Can you work these out from the model? Positions are in its coordinate system, mm. A direction names the side the tool comes from. Round coordinates to 2 decimals unless told otherwise and drop trailing zeros. Write each loop counter-clockwise with the first axis right and the second up, starting at its lowest first coordinate (ties: lowest second). Pieces come first, ordered by that corner, then holes. Notation, with made-up numbers: M -3.5,45 L 24.5,45 A22 ccw 24.5,71 Z; hole C 68,73.5 d10. An arc over 180 degrees is marked long. Answer as a JSON object with one key per item and string values. Group by question number.
1) Suppose I cut it at C-C, the plane z = 111. Write out the boundary of the cut face in (x, y).
2) Please list where these lines run through material, in increasing order: L1, parallel to Z at x = 22, y = 16.5; L2, parallel to X at y = 1, z = 9.5. Write a range as [from, to].
3) Suppose I cut it at B-B, the plane y = 0. Write out the boundary of the cut face in (x, z).
4) On a 3-axis mill with a long thin cutter (end or side, diameter ignored), from which of +Z, -Z, +X, -X, +Y, -Y can I reach the whole of each face in a straight line? I mean faces 1 (the flat face through (0, 0, 148)), 2 (the flat face through (37, 0, 131)), 3 (the cylindrical face through (32.07, 0.9, 120.14)), 4 (the flat face through (17, 1, 143)). Say none if no direction works.
5) Suppose I cut it at D-D, the plane z = 132.5. Write out the boundary of the cut face in (x, y), and give its area (3 significant figures).
6) Suppose I cut it at A-A, the plane x = 0. Write out the boundary of the cut face in (y, z), and give its area (3 significant figures).
7) I'm going to push flat-ended pins straight in: pin 1 Ø3 at (x, y) = (31, -3.5) entering from +Z; pin 2 Ø3 at (y, z) = (29.5, 97.5) entering from +X; pin 3 Ø10 at (y, z) = (-11.5, 65) entering from -X; pin 4 Ø5 at (x, y) = (-19.5, -1) entering from -Z. Where does each tip first touch, or does it pass through?
8) If we mould it in two halves opening along Z, with no side actions, what happens to faces 5 (the cylindrical face through (38, 0, 118)), 6 (the flat face through (27, 0, 123)), 7 (the cylindrical face through (-8.67, -39.05, 70.01)), 8 (the flat face through (-1, 1, 0))? For each: +Z half, -Z half, draft (parallel to the pull), parting line (faces both ways), or undercut.
from build123d import *

# Parameters (mm, degrees)
SKETCH_1_R          = 40
EXTRUDE_1_DEPTH     = 113
SKETCH_2_R          = 40
EXTRUDE_2_DEPTH     = 30
SKETCH_3_R          = 14
EXTRUDE_3_DEPTH     = 5
CUT_EXTRUDE_1_DEPTH = 34
SKETCH_6_R          = 3
CUT_EXTRUDE_2_DEPTH = 10
FILLET_1_R          = 1


with BuildPart() as part:
    # 草图1 → 凸台-拉伸1 (new body)
    with BuildSketch(Plane.XY):
        Circle(SKETCH_1_R)
    extrude(amount=EXTRUDE_1_DEPTH)

    # 草图2 → 凸台-拉伸2 (add)
    with BuildSketch(Plane.XY.offset(113)):
        Circle(SKETCH_2_R)
    extrude(amount=EXTRUDE_2_DEPTH)

    # 草图3 → 凸台-拉伸3 (add)
    with BuildSketch(Plane.XY.offset(143)):
        Circle(SKETCH_3_R)
    extrude(amount=EXTRUDE_3_DEPTH)

    # 草图5 → 切除-拉伸1 (cut)
    with BuildSketch(Plane(origin=(37, 0, 0), x_dir=(0, 0, -1), z_dir=(1, 0, 0))):
        with BuildLine():
            Line((-143, 0), (-143, -5))
            Line((-143, -5), (-123, -5))
            ThreePointArc((-123, -5), (-118, 0), (-123, 5))
            Line((-123, 5), (-143, 5))
            Line((-143, 5), (-143, 0))
        make_face()
    extrude(amount=CUT_EXTRUDE_1_DEPTH, mode=Mode.SUBTRACT)

    # 草图6 → 切除-拉伸2 (cut)
    with BuildSketch(Plane(origin=(37, 0, 0), x_dir=(0, 0, -1), z_dir=(1, 0, 0))):
        with Locations((-123, 0)):
            Circle(SKETCH_6_R)
    extrude(amount=-CUT_EXTRUDE_2_DEPTH, mode=Mode.SUBTRACT)

    # 圆角1
    fillet_1_edges = [part.edges().sort_by_distance(p)[0] for p in [
        (-40, 0, 143),
    ]]
    fillet(fillet_1_edges, radius=FILLET_1_R)


solid = part.part
Results:
{
 "1": {"outline": "C 0,0 d80"},
 "2": {"L1": "[0, 143]", "L2": "[-39.99, 39.99]"},
 "3": {"outline": "M -40,0 L 40,0 L 40,118 L 37,118 L 37,120 L 27,120 L 27,126 L 37,126 L 37,143 L 14,143 L 14,148 L -14,148 L -14,143 L -39,143 A1 ccw -40,142 Z"},
 "4": {"face 1": "+Z, +X, -X, +Y, -Y", "face 2": "+Z, +X", "face 3": "+X", "face 4": "+Z"},
 "5": {"outline": "M 37,-5 L 37,5 L 39.69,5 A40 ccw long 39.69,-5 Z", "area": "5,000 mm^2"},
 "6": {"outline": "M -40,0 L 40,0 L 40,142 A1 ccw 39,143 L 14,143 L 14,148 L -14,148 L -14,143 L -39,143 A1 ccw -40,142 Z", "area": "11,600 mm^2"},
 "7": {"pin 1": "z = 143", "pin 2": "x = 28.57", "pin 3": "x = -39.47", "pin 4": "z = 0"},
 "8": {"face 5": "+Z half", "face 6": "undercut", "face 7": "draft", "face 8": "-Z half"}
}
